```python
from build123d import *

# Parameters (mm, degrees)
SKETCH_1_R                   = 27.5
EXTRUDE_1_DEPTH              = 35
SKETCH_2_R                   = 15
EXTRUDE_2_DEPTH              = 5
HOLE_WIZARD_M5_1_D           = 4.2
HOLE_WIZARD_M5_1_CSINK_D     = 5.05
HOLE_WIZARD_M5_1_CSINK_ANGLE = 90
HOLE_WIZARD_M4_1_D           = 3.3
HOLE_WIZARD_M4_1_DEPTH       = 10.1
HOLE_WIZARD_M4_1_CSINK_D     = 4.05
HOLE_WIZARD_M4_1_CSINK_ANGLE = 90
HOLE_WIZARD_M4_1_TIP         = 0.991420021
FILLET_1_R                   = 0.25


with BuildPart() as part:
    # 草图1 → 凸台-拉伸1 (new body)
    with BuildSketch(Plane.XY):
        Circle(SKETCH_1_R)
    extrude(amount=EXTRUDE_1_DEPTH)

    # 草图2 → 凸台-拉伸2 (add)
    with BuildSketch(Plane.XY.offset(35)):
        Circle(SKETCH_2_R)
    extrude(amount=EXTRUDE_2_DEPTH)

    # M5 螺纹孔1 (through all)
    with Locations(Plane(origin=(0, 22.5, 0), x_dir=(-1, 0, 0), z_dir=(0, 0, -1))):
        with Locations((0, 0), (15.909902577, -6.590097423), (22.5, -22.5), (15.909902577, -38.409902577), (0, -45), (-15.909902577, -38.409902577), (-22.5, -22.5), (-15.909902577, -6.590097423)):
            CounterSinkHole(HOLE_WIZARD_M5_1_D / 2, HOLE_WIZARD_M5_1_CSINK_D / 2, counter_sink_angle=HOLE_WIZARD_M5_1_CSINK_ANGLE)

    # M4 螺纹孔1
    with Locations(Plane(origin=(0, 10, 40), x_dir=(1, 0, 0), z_dir=(0, 0, 1))):
        with Locations((0, 0), (8.660254038, -5), (8.660254038, -15), (0, -20), (-8.660254038, -15), (-8.660254038, -5)):
            CounterSinkHole(HOLE_WIZARD_M4_1_D / 2, HOLE_WIZARD_M4_1_CSINK_D / 2, depth=HOLE_WIZARD_M4_1_DEPTH, counter_sink_angle=HOLE_WIZARD_M4_1_CSINK_ANGLE)
            with Locations((0, 0, -(HOLE_WIZARD_M4_1_DEPTH + HOLE_WIZARD_M4_1_TIP / 2))):  # 118° drill point
                Cone(0, HOLE_WIZARD_M4_1_D / 2, HOLE_WIZARD_M4_1_TIP, mode=Mode.SUBTRACT)

    # 圆角1
    fillet_1_edges = [part.edges().sort_by_distance(p)[0] for p in [
        (-27.5, 0, 0),
        (-27.5, 0, 35),
        (-15, 0, 40),
    ]]
    fillet(fillet_1_edges, radius=FILLET_1_R)


solid = part.part
```
Here's how the part is built. I have some questions about the finished solid (model axes, mm). A direction names the side the tool comes from. Coordinates: 2 decimals unless noted, no trailing zeros.
1) Which directions (+Z, -Z, +X, -X, +Y, -Y) give clear straight access to the entire face, cutting with the end or side of a thin tool? Please do faces 4 (the face through (12, -12, 35)), 5 (the face through (-13.97, -16.71, 17.95)).
2) We'd pull the mould along X, two halves only. Please class faces 1 (the face through (0, 0, 40)), 2 (the face through (-14.985, 0.66, 37.342)), 3 (the face through (24.503, 0.631, 17.955)): +X half, -X half, draft (parallel to the pull), parting line (faces both ways), or undercut.
3) I need wall thicknesses on line 1 (Y direction, x = 0, z = 15); line 2 (Y direction, x = 0, z = 34); line 3 (X direction, y = -15.5, z = 3). Which ranges of each line are inside material? Lowest first, please.
4) Will these pins go through, and if not, where does the flat tip stop? pin 1 (5.5 mm diameter, centred on x = 0, y = 22.5, fed in from +Z); pin 2 (1.5 mm diameter, centred on y = 1.5, z = 22, fed in from -X); pin 3 (2.5 mm diameter, centred on x = 8.66, y = 5, fed in from +Z); pin 4 (4 mm diameter, centred on x = -22.5, y = 0, fed in from +Z).
5) Imagine slicing it at A-A on z = 23. State how many separate pieces and enclosed holes the cut face has, and give its area (4 significant figures).
Response values:
1. face 4: +Z
1. face 5: +Z, -Z
2. face 1: draft
2. face 2: parting line
2. face 3: undercut
3. line 1: y = -27.5 to -24.6, -20.4 to 20.4, 24.6 to 27.5
3. line 2: y = -27.5 to -24.6, -20.4 to -11.65, -8.35 to 8.35, 11.65 to 20.4, 24.6 to 27.5
3. line 3: x = -22.72 to -17.97, -13.85 to 13.85, 17.97 to 22.72
4. pin 1: stops at z = 35
4. pin 2: stops at x = -27.49
4. pin 3: stops at z = 29.66
4. pin 4: passes through
5. separate pieces: 1
5. enclosed holes: 8
5. area: 2,265 mm2
